Geometry check sheet. Reference: the model listing, model coordinates, mm. A direction names the side the tool comes from. Give positions to 0.01 mm unless a question says otherwise; leave off trailing zeros. Loops run counter-clockwise (first coordinate to the right, second up) from the corner with the lowest first, then second, coordinate; pieces in that order, holes last. Notation, with made-up numbers: (-33, 11) -> (-26, 11) arc R31 cw to (-26, 44) -> close; hole circle Ø9 at (21, 62.25). An arc over 180 degrees is marked (long way). Answer as a JSON object with one key per item and string values.
from build123d import *

# Parameters (mm, degrees)
F0_W         = 102
F0_H         = 62
F1_DEPTH     = 15
F2_R         = 1.5
F3_W         = 98.8
F3_H         = 58.8
F4_DEPTH     = 11
F5_W         = 7
F5_H         = 7
F5_R         = 1.15
F6_DEPTH     = 20
F7_T1_DEPTH  = 20
F7_T4_ANGLE  = 90
F7_T6_ANGLE  = 90
F7_T8_ANGLE  = 90
F7_T10_ANGLE = 90


# Not quite as in the source:
# - a fillet or chamfer that OpenCascade refuses, or shapes differently, is made with other operations: its cross-section is extruded or revolved along the edge and cut away or added
# - a feature names something its author has since deleted; it is built from what else it names


with BuildPart() as f1:
    # F0 (on Right) → F1 (new body)
    with BuildSketch(Plane.YZ):
        with Locations((-6.9849695861, 0.5)):
            Rectangle(F0_W, F0_H)
    extrude(amount=-F1_DEPTH)

    # F2
    f2_edges = [f1.edges().sort_by_distance(p)[0] for p in [
        (-15, -6.98497, 31.5),
        (-15, -57.98497, 0.5),
        (-15, -6.98497, -30.5),
        (-15, 44.01503, 0.5),
    ]]
    fillet(f2_edges, radius=F2_R)

    # F3 (on face) → F4 (cut)
    with BuildSketch(Plane.YZ):
        with Locations((-6.9849695861, 0.5)):
            Rectangle(F3_W, F3_H)
    extrude(amount=-F4_DEPTH, mode=Mode.SUBTRACT)

    # F5 (on face) → F6 (join)
    with BuildSketch(Plane.YZ.offset(-11)):
        with Locations((-52.8849695861, -25.4)):
            Rectangle(F5_W, F5_H)
        with Locations((-52.1849695861, -24.9)):
            Circle(F5_R, mode=Mode.SUBTRACT)
        with Locations((38.9150304139, -25.4)):
            Rectangle(F5_W, F5_H)
        with Locations((38.2150304139, -24.9)):
            Circle(F5_R, mode=Mode.SUBTRACT)
        with Locations((38.9150304139, 26.4)):
            Rectangle(F5_W, F5_H)
        with Locations((38.2150304139, 25.9)):
            Circle(F5_R, mode=Mode.SUBTRACT)
        with Locations((-52.8849695861, 26.4)):
            Rectangle(F5_W, F5_H)
        with Locations((-52.1849695861, 25.9)):
            Circle(F5_R, mode=Mode.SUBTRACT)
    extrude(amount=F6_DEPTH)

    # F7: fillet of radius 2 on 4 edges, made by hand

    # F7_s2 → F7_t1 (cut)
    with BuildSketch(Plane.YZ.offset(-15)):
        with BuildLine():
            ThreePointArc((-55.9849695861, -30.5), (-57.3991831485, -29.9142135624), (-57.9849695861, -28.5))
            Line((-57.9849695861, -28.5), (-57.9849695861, -30.5))
            Line((-57.9849695861, -30.5), (-55.9849695861, -30.5))
        make_face()
        with BuildLine():
            ThreePointArc((-57.9849695861, 29.5), (-57.3991831485, 30.9142135624), (-55.9849695861, 31.5))
            Line((-55.9849695861, 31.5), (-57.9849695861, 31.5))
            Line((-57.9849695861, 31.5), (-57.9849695861, 29.5))
        make_face()
        with BuildLine():
            ThreePointArc((44.0150304139, 29.5), (43.4292439762, 30.9142135624), (42.0150304139, 31.5))
            Line((42.0150304139, 31.5), (44.0150304139, 31.5))
            Line((44.0150304139, 31.5), (44.0150304139, 29.5))
        make_face()
        with BuildLine():
            ThreePointArc((42.0150304139, -30.5), (43.4292439762, -29.9142135624), (44.0150304139, -28.5))
            Line((44.0150304139, -28.5), (44.0150304139, -30.5))
            Line((44.0150304139, -30.5), (42.0150304139, -30.5))
        make_face()
    extrude(amount=F7_T1_DEPTH, mode=Mode.SUBTRACT)

    # F7_s3 → F7_t4 (revolve, cut)
    with BuildSketch(Plane.XY.offset(-28.5)):
        with BuildLine():
            ThreePointArc((-15, 42.5150304139), (-14.5606601718, 43.5756905856), (-13.5, 44.0150304139))
            Line((-13.5, 44.0150304139), (-15, 44.0150304139))
            Line((-15, 44.0150304139), (-15, 42.5150304139))
        make_face()
    revolve(axis=Axis((-15, 42.0150304139, -28.5), (-1, 0, 0)), revolution_arc=F7_T4_ANGLE, mode=Mode.SUBTRACT)

    # F7_s5 → F7_t6 (revolve, cut)
    with BuildSketch(Plane.XZ.offset(-42.0150304139)):
        with BuildLine():
            ThreePointArc((-15, 30), (-14.5606601718, 31.0606601718), (-13.5, 31.5))
            Line((-13.5, 31.5), (-15, 31.5))
            Line((-15, 31.5), (-15, 30))
        make_face()
    revolve(axis=Axis((-15, 42.0150304139, 29.5), (-1, 0, 0)), revolution_arc=F7_T6_ANGLE, mode=Mode.SUBTRACT)

    # F7_s7 → F7_t8 (revolve, cut)
    with BuildSketch(Plane.XY.offset(29.5)):
        with BuildLine():
            ThreePointArc((-15, -56.4849695861), (-14.5606601718, -57.5456297579), (-13.5, -57.9849695861))
            Line((-13.5, -57.9849695861), (-15, -57.9849695861))
            Line((-15, -57.9849695861), (-15, -56.4849695861))
        make_face()
    revolve(axis=Axis((-15, -55.9849695861, 29.5), (-1, 0, 0)), revolution_arc=F7_T8_ANGLE, mode=Mode.SUBTRACT)

    # F7_s9 → F7_t10 (revolve, cut)
    with BuildSketch(Plane.XZ.offset(55.9849695861)):
        with BuildLine():
            ThreePointArc((-15, -29), (-14.5606601718, -30.0606601718), (-13.5, -30.5))
            Line((-13.5, -30.5), (-15, -30.5))
            Line((-15, -30.5), (-15, -29))
        make_face()
    revolve(axis=Axis((-15, -55.9849695861, -28.5), (-1, 0, 0)), revolution_arc=F7_T10_ANGLE, mode=Mode.SUBTRACT)


solid = f1.part
1) Draft check along Y on faces 6 (the face through (4, -56.385, 26)), 7 (the face through (4, 42.415, -25)), 8 (the face through (-11, 38, -25)). Enter one of: pulls with the +Y half, pulls with the -Y half, needs draft (parallel to the pull), parting line crosses it, or undercut.
Geometry check:
{"face 6": "pulls with the -Y half", "face 7": "pulls with the +Y half", "face 8": "undercut"}
2) Section check C-C on y = -31. Record the cut outline in (x, z), plus the area to 3 significant figures.
Geometry check:
{"outline": "(-15, -29) arc R1.5 ccw to (-13.5, -30.5) -> (0, -30.5) -> (0, -28.9) -> (-11, -28.9) -> (-11, 29.9) -> (0, 29.9) -> (0, 31.5) -> (-13.5, 31.5) arc R1.5 ccw to (-15, 30) -> close", "area": "282 mm2"}
3) Section check B-B on z = -24.9. Record the cut outline in (x, y), plus the area to 3 significant figures.
Geometry check:
{"outline": "(-15, -56.48) arc R1.5 ccw to (-13.5, -57.98) -> (0, -57.98) -> (0, -56.38) -> (9, -56.38) -> (9, -53.33) -> (-11, -53.33) -> (-11, -51.03) -> (9, -51.03) -> (9, -49.38) -> (-11, -49.38) -> (-11, 35.42) -> (9, 35.42) -> (9, 37.07) -> (-11, 37.07) -> (-11, 39.37) -> (9, 39.37) -> (9, 42.42) -> (0, 42.42) -> (0, 44.02) -> (-13.5, 44.02) arc R1.5 ccw to (-15, 42.52) -> close", "area": "630 mm2"}
4) Depth check by flat-ended pin: P1, Ø10, axis at y = -22.5, z = -19.5, coming from the +X side; P2, Ø2, axis at x = 3.5, z = 25.5, coming from the -Y side; P3, Ø2, axis at x = 3, z = -24.5, coming from the +Y side; P4, Ø3, axis at x = 1, y = -19, coming from the -Z side. Enter the tip coordinate at first touch or a pass-through.
Geometry check:
{"P1": "stops at x = -11", "P2": "stops at y = -56.38", "P3": "stops at y = 42.42", "P4": "stops at z = -30.5"}
5) Tool access check on faces 1 (the face through (-11, -52, -25)), 2 (the face through (4, -56.385, -25)), 3 (the face through (4, 39, -28.9)), 4 (the face through (9, 40, 26)), 5 (the face through (4, -53, 29.9)). Record the directions out of +Z, -Z, +X, -X, +Y, -Y that give a thin tool (end or side, any length) a straight path to the whole face; none if there is none.
Geometry check:
{"face 1": "+X", "face 2": "+Z, -Z, +X, -Y", "face 3": "-Z, +X, +Y, -Y", "face 4": "+Z, -Z, +X, +Y, -Y", "face 5": "+Z, +X, +Y, -Y"}
6) Section check A-A on x = -1.75. Record the cut outline in (y, z), plus the area to 3 significant figures.
Geometry check:
{"outline": "(-57.98, -28.5) arc R2 ccw to (-55.98, -30.5) -> (42.02, -30.5) arc R2 ccw to (44.02, -28.5) -> (44.02, 29.5) arc R2 ccw to (42.02, 31.5) -> (-55.98, 31.5) arc R2 ccw to (-57.98, 29.5) -> close; hole (-56.38, -21.9) -> (-49.38, -21.9) -> (-49.38, -28.9) -> (35.42, -28.9) -> (35.42, -21.9) -> (42.42, -21.9) -> (42.42, 22.9) -> (35.42, 22.9) -> (35.42, 29.9) -> (-49.38, 29.9) -> (-49.38, 22.9) -> (-56.38, 22.9) -> close; hole circle Ø2.3 at (-52.18, -24.9); hole circle Ø2.3 at (-52.18, 25.9); hole circle Ø2.3 at (38.22, -24.9); hole circle Ø2.3 at (38.22, 25.9)", "area": "691 mm2"}
7) Material ranges on line 1 along Z through (x, y) = (-5, -52); line 2 along Z through (x, y) = (-1, -19.5); line 3 along Y through (x, z) = (-0.75, -7), recorded low to high. Write a range as from..to.
Geometry check:
{"line 1": "z = -30.5..-26.04, -23.76..-21.9, 22.9..24.76, 27.04..31.5", "line 2": "z = -30.5..-28.9, 29.9..31.5", "line 3": "y = -57.98..-56.38, 42.42..44.02"}
8) Section check D-D on z = -2. Record the cut outline in (x, y), plus the area to 3 significant figures.
Geometry check:
{"outline": "(-15, -56.48) arc R1.5 ccw to (-13.5, -57.98) -> (0, -57.98) -> (0, -56.38) -> (-11, -56.38) -> (-11, 42.42) -> (0, 42.42) -> (0, 44.02) -> (-13.5, 44.02) arc R1.5 ccw to (-15, 42.52) -> close", "area": "442 mm2"}
